Here's how the part is built. I have some questions about the finished solid (model axes, mm). A direction names the side the tool comes from. Coordinates: 2 decimals unless noted, no trailing zeros. Write each loop counter-clockwise with the first axis right and the second up, starting at its lowest first coordinate (ties: lowest second). Pieces come first, ordered by that corner, then holes. Notation, with made-up numbers: (18, -24.75) -> (69, -24.75) arc R29 ccw to (69, 9.25) -> close; hole circle Ø10 at (17.25, -24.5). An arc over 180 degrees is marked (long way). Use a Markdown table: item, result. Add a question column.
Item 1: On a 3-axis mill with a long thin cutter (end or side, diameter ignored), from which of +Z, -Z, +X, -X, +Y, -Y can I reach the whole of each face in a straight line? I mean faces 1 (the flat face through (54, 118, 4)), 2 (the flat face through (110, 59, 2)). Say none if no direction works.
Item 2: Imagine slicing it at D-D, the plane x = 90.5. Write out the boundary of the cut face in (y, z), and give its area (3 significant figures).
Item 3: Imagine slicing it at B-B, the plane x = 32. Write out the boundary of the cut face in (y, z), and give its area (3 significant figures).
Item 4: Imagine slicing it at A-A, the plane y = 60. Write out the boundary of the cut face in (x, z), and give its area (3 significant figures).
Item 5: If I drill on line 1 along Y through (x, z) = (32, 0.85); line 2 along X through (y, z) = (60, 0.6); line 3 along X through (y, z) = (101.5, 0.9), over which ranges is the centre line in solid material (lowest first)? Write a range as from..to.
Item 6: Imagine slicing it at C-C, the plane y = 101.5. Write out the boundary of the cut face in (x, z).
Item 7: Will this pin go through, and if not, where does the flat tip stop? pin 1 Ø3 at (x, y) = (75, 98.5) entering from +Z.
Item 8: If we mould it in two halves opening along Y, with no side actions, what happens to faces 3 (the flat face through (1.8, 86.9, 5)), 4 (the cylindrical face through (97.805, 58.513, 0.986)), 5 (the flat face through (54, 0, 2)), 6 (the flat face through (54, 120, 2))? For each: pulls with the +Y half, pulls with the -Y half, needs draft (parallel to the pull), parting line crosses it, or undercut.
```python
from build123d import *

# Parameters (mm, degrees)
SKETCH_W        = 110
SKETCH_H        = 120
SKETCH_R        = 2.5
PAD_DEPTH       = 5
SKETCH001_W     = 106
SKETCH001_H     = 116
POCKET_DEPTH    = 3
SKETCH002_R     = 1.5
SKETCH002_W     = 33
SKETCH002_H     = 67
SKETCH002_W_2   = 30
SKETCH002_H_2   = 73.5
POCKET001_DEPTH = 5.001


with BuildPart() as part:
    # Sketch → Pad (new body)
    with BuildSketch(Plane.XY):
        with Locations((55, 60)):
            Rectangle(SKETCH_W, SKETCH_H)
        with Locations((32, 101.5)):
            Circle(SKETCH_R, mode=Mode.SUBTRACT)
        with Locations((78, 101.5)):
            Circle(SKETCH_R, mode=Mode.SUBTRACT)
        with Locations((32, 18.5)):
            Circle(SKETCH_R, mode=Mode.SUBTRACT)
        with Locations((78, 18.5)):
            Circle(SKETCH_R, mode=Mode.SUBTRACT)
    extrude(amount=PAD_DEPTH)

    # Sketch001 → Pocket (cut)
    with BuildSketch(Plane.XY.offset(5)):
        with Locations((55, 60)):
            Rectangle(SKETCH001_W, SKETCH001_H)
    extrude(amount=-POCKET_DEPTH, mode=Mode.SUBTRACT)

    # Sketch002 → Pocket001 (cut, through all)
    with BuildSketch(Plane(origin=(0, 0, 0), x_dir=(1, 0, 0), z_dir=(0, 0, -1))):
        with Locations((58, -60)):
            Circle(SKETCH002_R)
        with Locations((98, -60)):
            Circle(SKETCH002_R)
        with Locations((32, -60)):
            Rectangle(SKETCH002_W, SKETCH002_H)
        with Locations((78, -59.75)):
            Rectangle(SKETCH002_W_2, SKETCH002_H_2)
    extrude(amount=-POCKET001_DEPTH, mode=Mode.SUBTRACT)


solid = part.part
```
Ans:
| question | item | result |
|---|---|---|
| 1 | face 1 | +Z |
| 1 | face 2 | +Z, -Z, +X, +Y, -Y |
| 2 | outline | (0, 0) -> (23, 0) -> (23, 2) -> (2, 2) -> (2, 5) -> (0, 5) -> close; (96.5, 0) -> (120, 0) -> (120, 5) -> (118, 5) -> (118, 2) -> (96.5, 2) -> close |
| 2 | area | 105 mm^2 |
| 3 | outline | (0, 0) -> (16, 0) -> (16, 2) -> (2, 2) -> (2, 5) -> (0, 5) -> close; (21, 0) -> (26.5, 0) -> (26.5, 2) -> (21, 2) -> close; (93.5, 0) -> (99, 0) -> (99, 2) -> (93.5, 2) -> close; (104, 0) -> (120, 0) -> (120, 5) -> (118, 5) -> (118, 2) -> (104, 2) -> close |
| 3 | area | 98.0 mm^2 |
| 4 | outline | (0, 0) -> (15.5, 0) -> (15.5, 2) -> (2, 2) -> (2, 5) -> (0, 5) -> close; (48.5, 0) -> (56.5, 0) -> (56.5, 2) -> (48.5, 2) -> close; (59.5, 0) -> (63, 0) -> (63, 2) -> (59.5, 2) -> close; (93, 0) -> (96.5, 0) -> (96.5, 2) -> (93, 2) -> close; (99.5, 0) -> (110, 0) -> (110, 5) -> (108, 5) -> (108, 2) -> (99.5, 2) -> close |
| 4 | area | 94.0 mm^2 |
| 5 | line 1 | y = 0..16, 21..26.5, 93.5..99, 104..120 |
| 5 | line 2 | x = 0..15.5, 48.5..56.5, 59.5..63, 93..96.5, 99.5..110 |
| 5 | line 3 | x = 0..29.5, 34.5..75.5, 80.5..110 |
| 6 | outline | (0, 0) -> (29.5, 0) -> (29.5, 2) -> (2, 2) -> (2, 5) -> (0, 5) -> close; (34.5, 0) -> (75.5, 0) -> (75.5, 2) -> (34.5, 2) -> close; (80.5, 0) -> (110, 0) -> (110, 5) -> (108, 5) -> (108, 2) -> (80.5, 2) -> close |
| 7 | pin 1 | stops at z = 2 |
| 8 | face 3 | needs draft |
| 8 | face 4 | undercut |
| 8 | face 5 | pulls with the -Y half |
| 8 | face 6 | pulls with the +Y half |
